from build123d import *

# Parameters (mm, degrees)
SKETCH1_W           = 91.58
SKETCH1_H           = 10
BOSS_EXTRUDE1_DEPTH = 53
SKETCH2_R           = 1.75
CUT_EXTRUDE1_DEPTH  = 71.75114204
SKETCH4_W           = 15
SKETCH4_H           = 25
CUT_EXTRUDE3_DEPTH  = 8
SKETCH5_R           = 2.25
CUT_EXTRUDE4_DEPTH  = 17
SKETCH7_R           = 3.5
CUT_EXTRUDE5_DEPTH  = 4.5
FILLET1_R           = 2.5


with BuildPart() as part:
    # Sketch1 → Boss-Extrude1 (new body)
    with BuildSketch(Plane(origin=(0, 0, 0), x_dir=(1, 0, 0), z_dir=(0, 1, 0))):
        Rectangle(SKETCH1_W, SKETCH1_H)
    extrude(amount=BOSS_EXTRUDE1_DEPTH)

    # Sketch2 → Cut-Extrude1 (cut, through all)
    with BuildSketch(Plane.XY.offset(5)):
        with Locations((33.464, 4.763)):
            Circle(SKETCH2_R)
        with Locations((-16.828, 4.382)):
            Circle(SKETCH2_R)
    extrude(amount=-CUT_EXTRUDE1_DEPTH, mode=Mode.SUBTRACT)

    # Sketch4 → Cut-Extrude3 (cut)
    with BuildSketch(Plane(origin=(0, 0, -5), x_dir=(-1, 0, 0), z_dir=(0, 0, -1))):
        with Locations((22.5, 35.5)):
            Rectangle(SKETCH4_W, SKETCH4_H)
        with Locations((-22.5, 35.5)):
            Rectangle(SKETCH4_W, SKETCH4_H)
    extrude(amount=-CUT_EXTRUDE3_DEPTH, mode=Mode.SUBTRACT)

    # Sketch5 → Cut-Extrude4 (cut)
    with BuildSketch(Plane(origin=(0, 53, 0), x_dir=(1, 0, 0), z_dir=(0, 1, 0))):
        with Locations(Location((22.5, 1, 0), (0, 0, 270))):
            Circle(SKETCH5_R)
        with Locations(Location((-22.5, 1, 0), (0, 0, 270))):
            Circle(SKETCH5_R)
    extrude(amount=-CUT_EXTRUDE4_DEPTH, mode=Mode.SUBTRACT)

    # Sketch7 → Cut-Extrude5 (cut)
    with BuildSketch(Plane.XY.offset(5)):
        with Locations((33.464, 4.763)):
            Circle(SKETCH7_R)
        with Locations((-16.828, 4.382)):
            Circle(SKETCH7_R)
    extrude(amount=-CUT_EXTRUDE5_DEPTH, mode=Mode.SUBTRACT)

    # Sketch9 → M3 Tapped Hole1 (revolve, cut)
    with BuildSketch(Plane(origin=(-45.79, 7, 0), x_dir=(0, 0, 1), z_dir=(0, 1, 0))):
        Polygon((0, 0), (0, 8.251075774), (1.25, 7.5), (1.25, 0), align=None)
    m3_tapped_hole1 = revolve(axis=Axis((-52.14, 7, 0), (1, 0, 0)), mode=Mode.SUBTRACT)

    # Mirror1: M3 Tapped Hole1 across plane
    add(m3_tapped_hole1.mirror(Plane(origin=(0, 0, 0), x_dir=(0, 0, 1), z_dir=(1, 0, 0))), mode=Mode.SUBTRACT)

    # Fillet1
    fillet1_edges = [part.edges().sort_by_distance(p)[0] for p in [
        (-30, 48, -1),
        (-30, 23, -1),
        (-15, 23, -1),
        (-15, 48, -1),
        (15, 48, -1),
        (15, 23, -1),
        (30, 23, -1),
        (30, 48, -1),
    ]]
    fillet(fillet1_edges, radius=FILLET1_R)


solid = part.part
Design review of the part built by this model. Coordinates are the model's own, in mm. A direction names the side the tool comes from. Give positions to 0.01 mm unless a question says otherwise; leave off trailing zeros. Loops run counter-clockwise (first coordinate to the right, second up) from the corner with the lowest first, then second, coordinate; pieces in that order, holes last. Notation, with made-up numbers: (38.5, 0) - (90.5, 0) arc R27 ccw to (90.5, 26) - close; hole circle Ø1 at (57.25, -22.75). An arc over 180 degrees is marked (long way). Use CSV: the item, a comma, the result in double quotes. Start each with the question number.
1. Wall thickness on L1, parallel to X at y = 28, z = -3; L2, parallel to Y at x = 42.25, z = 0; L3, parallel to X at y = 51, z = 0.25: over which ranges is each line inside the solid? List them lowest first.
2. Machinability: for faces 1 (the flat face through (32, 6, 0.5)), 2 (the flat face through (15, 35, -1)), 3 (the cylindrical face through (20.304, 50.535, -1.488)), which of the approach directions +Z, -Z, +X, -X, +Y, -Y give a long, thin tool a straight path to every point of the face, cutting with its end or side? Answer none if there is none.
3. Insertion check: P1, Ø2.5, axis at x = 22, z = -0.5, coming from the +Y side; P2, Ø4, axis at x = -21, z = 0, coming from the -Y side; P3, Ø7.5, axis at x = -24, y = 33.5, coming from the -Z side; P4, Ø5.5, axis at x = 34, y = 5, coming from the +Z side. Each pin has a flat end and moves straight along its axis. Give the tip position at first contact, or say it passes through.
4. Draft analysis for pull direction Y (two halves, no side actions). For faces 4 (the flat face through (-45.79, 26, 0)), 5 (the flat face through (23, 36, 3)), state which applies: released by +Y, released by -Y, zero draft, split by the parting line, or undercut.
5. Add section B-B (y = 42.5). State the section outline as (x, z) points.
6. Add section A-A (x = -22.5). State the section outline as (y, z) points, plus the area to 4 significant figures.
Results found:
1,L1,"x = -45.79 to -30, -15 to 15, 30 to 45.79"
1,L2,"y = 0 to 5.75, 8.25 to 53"
1,L3,"x = -45.79 to -24.37, -20.63 to 20.63, 24.37 to 45.79"
2,face 1,"+Z"
2,face 2,"-Z"
2,face 3,"+Y"
3,P1,"stops at y = 23"
3,P2,"stops at y = 0"
3,P3,"stops at z = 3"
3,P4,"stops at z = 0.5"
4,face 4,"zero draft"
4,face 5,"undercut"
5,outline,"(-45.79, -5) - (-30, -5) - (-30, 3) - (-15, 3) - (-15, -5) - (15, -5) - (15, 3) - (30, 3) - (30, -5) - (45.79, -5) - (45.79, 5) - (-45.79, 5) - close"
6,outline,"(0, -5) - (23, -5) - (23, 3) - (48, 3) - (48, 1.25) - (53, 1.25) - (53, 5) - (0, 5) - close; (48, -5) - (53, -5) - (53, -3.25) - (48, -3.25) - close"
6,area,"307.5 mm²"
